Autodesk Inventor part; units mm, degrees
ref_plane "YZ Plane" through (0, 0, 0) normal (1, 0, 0) x (0, 1, 0)
ref_plane "XZ Plane" through (0, 0, 0) normal (0, 1, 0) x (-1, 0, 0)
ref_plane "XY Plane" through (0, 0, 0) normal (0, 0, 1) x (1, 0, 0)
sketch "Skizze1" plane through (0, 0, 0) normal (1, 0, 0) x (0, 1, 0)
  line L0 (9, 16) -> (9, -16)
  line L1 (9, -16) -> (7.5, -16)
  line L2 (7.5, -16) -> (7.5, -1)
  line L3 (7.5, -1) -> (-7.5, -1)
  line L4 (-7.5, -1) -> (-7.5, -16)
  line L5 (-7.5, -16) -> (-9, -16)
  line L6 (-9, -16) -> (-9, 16)
  line L7 (-9, 16) -> (-7.5, 16)
  line L8 (-7.5, 16) -> (-7.5, 1)
  line L9 (-7.5, 1) -> (7.5, 1)
  line L10 (9, 16) -> (7.5, 16)
  line L11 (7.5, 16) -> (7.5, 1)
  line L12 (0, 0) -> (9, 0) construction
  line L13 (0, 0) -> (-9, 0) construction
  line L14 (0, 0) -> (0, 16) construction
  line L15 (0, 0) -> (0, -16) construction
  dimension "d0" = 2
  dimension "d1" = 1.5
  dimension "d2" = 32
  dimension "d3" = 18
extrude "Extrusion1" add sketch "Skizze1" along normal mid plane 1000
sketch "Skizze2" plane through (-500, -9, 16) normal (0, 1, 0) x (1, 0, 0)
  line L0 (985, 23.5) -> (985, 8.5)
  line L1 (15, 23.5) -> (15, 8.5)
  line L2 (15, 16) -> (0, 16)
  line L3 (0, 0) -> (0, 32)
  line L4 (1000, 32) -> (1000, 0)
  line L5 (985, 16) -> (1000, 16)
  point P0 (500, 16)
  dimension "d6" = 15
  dimension "d8" = 15
  dimension "d9" = 15
  dimension "d17" = 8.5
  dimension "d18" = 15
hole "Bohrung1" at (485, -9, -7.5) at (485, -9, 7.5) at (-485, -9, -7.5) at (-485, -9, 7.5) direction (0, 1, 0) diameter 5 depth 1.5
properties part number "Träger" material "Aluminium 6061, Träger"
Geometry: final body of the model. Coordinates: model frame, mm. Coordinates: 2 decimals unless noted, no trailing zeros. Order: outer loops, then holes, each group sorted by start corner. A loop starts at its lowest first (then second) coordinate and runs counter-clockwise, first axis right, second up. Notation, with made-up numbers: M 9.5,71.5 L 35.5,71.5 A28 ccw 35.5,96.5 Z; hole C 53.25,-18.75 d1. An arc over 180 degrees is marked long. Answer as CSV lines item,"result".
Q1. First-contact query: P1, Ø4, axis at x = 485, z = -7.5, coming from the -Y side; P2, Ø2, axis at x = 231.5, y = 3, coming from the -Z side; P3, Ø3, axis at x = -206, y = 2.5, coming from the +Z side. Flat tips, straight axial feed; report the tip coordinate or a pass-through.
Answers:
P1,"stops at y = 7.5"
P2,"stops at z = -1"
P3,"stops at z = 1"
Q2. Line query: probe 1 along Z at (x, y) = (485, -8.65); probe 2 along X at (y, z) = (-8.4, -7.5); probe 3 along Y at (x, z) = (346, 13). Output: solid intervals per line, ascending. Write a range as [from, to].
Answers:
probe 1,"z = [-16, -10], [-5, 5], [10, 16]"
probe 2,"x = [-500, -487.5], [-482.5, 482.5], [487.5, 500]"
probe 3,"y = [-9, -7.5], [7.5, 9]"
Q3. Section A-A on x = -198. Return the cut outline in (y, z).
Answers:
outline,"M -9,-16 L -7.5,-16 L -7.5,-1 L 7.5,-1 L 7.5,-16 L 9,-16 L 9,16 L 7.5,16 L 7.5,1 L -7.5,1 L -7.5,16 L -9,16 Z"
Q4. Section B-B on y = 0.75. Return the cut outline in (x, z), and give its area (3 significant figures).
Answers:
outline,"M -500,-1 L 500,-1 L 500,1 L -500,1 Z"
area,"2,000 mm^2"
